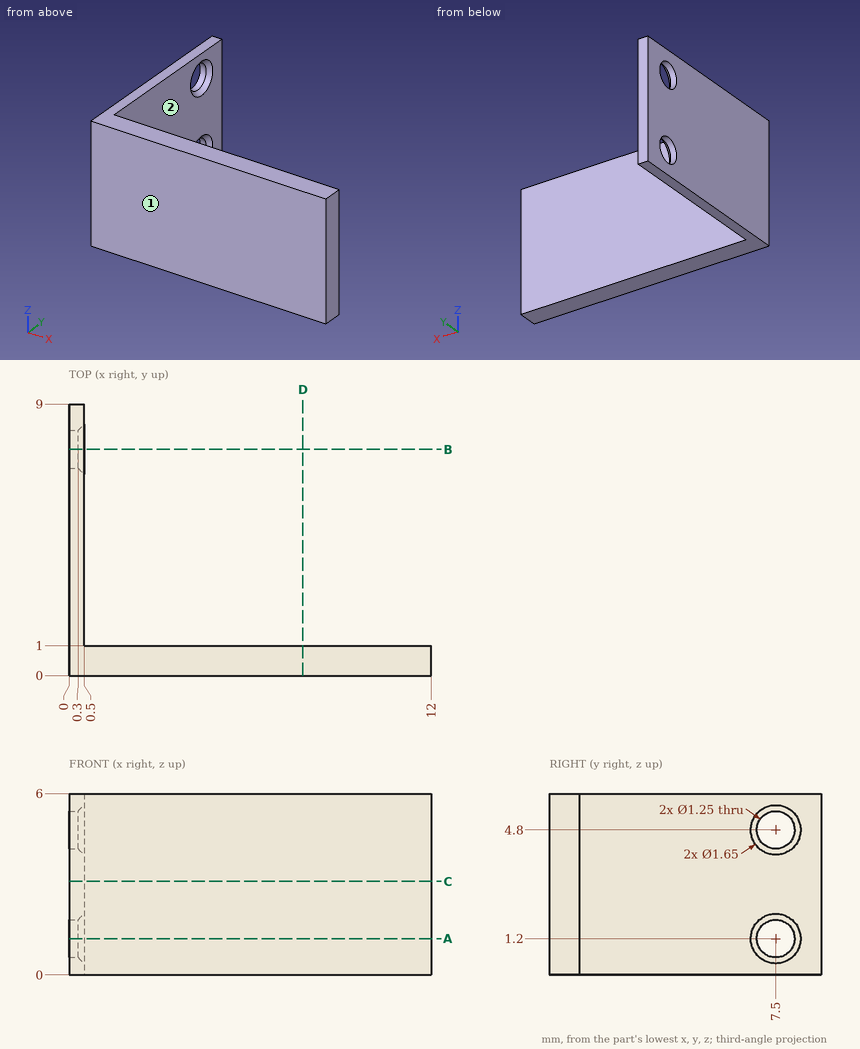
Could you check a few things on this drawing? It's one solid part, dimensions in mm from its lowest x, y, z. A direction names the side the tool comes from. Give positions to 0.01 mm unless a question says otherwise; leave off trailing zeros. Order: outer loops, then holes, each group sorted by start corner. A loop starts at its lowest first (then second) coordinate and runs counter-clockwise, first axis right, second up. Notation, with made-up numbers: (-18.75, 15.5) - (4.25, 15.5) arc R22 ccw to (4.25, 51.5) - close; hole circle Ø10 at (2.5, -35). An arc over 180 degrees is marked (long way). Return JSON: item names as keys, results as strings. Group by question number.
Q1. Please list where these lines run through material, in increasing order: line 1 along Z through (x, y) = (0.15, 7.5) (3 decimals); line 2 along Y through (x, z) = (0.15, 1.2) (3 decimals); line 3 along Y through (x, z) = (7.5, 1.2). Write a range as [from, to].
Q2. Suppose I cut it at D-D, the plane x = 7.75. Please give me the cut outline in (y, z).
Q3. Suppose I cut it at A-A, the plane z = 1.2. Please give me the cut outline in (x, y) (3 decimals).
Q4. Will these pins go through, and if not, where does the flat tip stop? pin 1 Ø2 at (y, z) = (7, 1) entering from +X; pin 2 Ø1.4 at (y, z) = (7.5, 4.8) entering from +X (3 decimals); pin 3 Ø2 at (x, z) = (5, 4) entering from +Y.
Q5. Suppose I cut it at C-C, the plane z = 3.1. Please give me the cut outline in (x, y).
Q6. Suppose I cut it at B-B, the plane y = 7.5. Please give me the cut outline in (x, z) (3 decimals).
Q7. Which directions (+Z, -Z, +X, -X, +Y, -Y) give clear straight access to the entire face, cutting with the end or side of a thin tool? Please do the marked faces 1 and 2.
Resolved:
{
 "1": {"line 1": "z = [0, 0.575], [1.825, 4.175], [5.425, 6]", "line 2": "y = [0, 6.875], [8.125, 9]", "line 3": "y = [0, 1]"},
 "2": {"outline": "(0, 0) - (1, 0) - (1, 6) - (0, 6) - close"},
 "3": {"outline": "(0, 0) - (12, 0) - (12, 1) - (0.5, 1) - (0.5, 6.675) - (0.3, 6.875) - (0, 6.875) - close; (0, 8.125) - (0.3, 8.125) - (0.5, 8.325) - (0.5, 9) - (0, 9) - close"},
 "4": {"pin 1": "stops at x = 0.5", "pin 2": "stops at x = 0.375", "pin 3": "stops at y = 1"},
 "5": {"outline": "(0, 0) - (12, 0) - (12, 1) - (0.5, 1) - (0.5, 9) - (0, 9) - close"},
 "6": {"outline": "(0, 0) - (0.5, 0) - (0.5, 0.375) - (0.3, 0.575) - (0, 0.575) - close; (0, 1.825) - (0.3, 1.825) - (0.5, 2.025) - (0.5, 3.975) - (0.3, 4.175) - (0, 4.175) - close; (0, 5.425) - (0.3, 5.425) - (0.5, 5.625) - (0.5, 6) - (0, 6) - close"},
 "7": {"face 1": "+Z, -Z, +X, -X, -Y", "face 2": "+Z, -Z, +X, +Y"}
}
